from build123d import *

# Parameters (mm, degrees)
BOSS_EXTRUDE1_DEPTH        = 50.8
CUT_EXTRUDE1_REACH         = 65.5
SKETCH2_R                  = 12.7
F_10_32_TAPPED_HOLE1_D     = 4.0386
F_10_32_TAPPED_HOLE1_DEPTH = 6.35
F_10_32_TAPPED_HOLE2_D     = 4.0386
F_10_32_TAPPED_HOLE2_DEPTH = 6.35


with BuildPart() as part:
    # Sketch1 → Boss-Extrude1 (new body)
    with BuildSketch(Plane.XY):
        Polygon((0, 0), (63.5, 0), (63.5, -63.5), (57.15, -63.5), (57.15, -6.35), (0, -6.35), align=None)
    extrude(amount=BOSS_EXTRUDE1_DEPTH)

    # Sketch2 → Cut-Extrude1 (cut, up to next)
    with BuildSketch(Plane(origin=(63.5, 0, 0), x_dir=(0, 0, -1), z_dir=(1, 0, 0)), mode=Mode.PRIVATE) as cut_extrude1_sk1:
        with Locations((-25.4, -31.75)):
            Circle(SKETCH2_R)
    cut_extrude1_tool1 = extrude(cut_extrude1_sk1.sketch, amount=-CUT_EXTRUDE1_REACH, mode=Mode.PRIVATE) & part.part
    add(cut_extrude1_tool1.solids().sort_by_distance((63.5, -31.75, 25.4))[0], mode=Mode.SUBTRACT)

    # #10-32 Tapped Hole1
    with Locations(Plane(origin=(63.5, 0, 0), x_dir=(0, 0, -1), z_dir=(1, 0, 0))):
        with Locations((-34.925, -50.8), (-15.875, -50.8), (-34.925, -12.7), (-15.875, -12.7)):
            Hole(F_10_32_TAPPED_HOLE1_D / 2, depth=F_10_32_TAPPED_HOLE1_DEPTH)

    # #10-32 Tapped Hole2
    with Locations(Plane(origin=(0, 0, 0), x_dir=(1, 0, 0), z_dir=(0, 1, 0))):
        with Locations((47.625, -44.45), (31.75, -38.1), (15.875, -44.45)):
            Hole(F_10_32_TAPPED_HOLE2_D / 2, depth=F_10_32_TAPPED_HOLE2_DEPTH)


solid = part.part
The listing builds one solid part. Answer for the finished solid, in the listing's coordinates (mm). A direction names the side the tool comes from. Round coordinates to 2 decimals unless told otherwise and drop trailing zeros. Order: outer loops, then holes, each group sorted by start corner. A loop starts at its lowest first (then second) coordinate and runs counter-clockwise, first axis right, second up. Notation, with made-up numbers: M 80.25,72 L 118.25,72 A18 ccw 118.25,84 Z; hole C -16.75,9 d3. An arc over 180 degrees is marked long. Answer in a Markdown table with one row per item. Add a question column.
1) The part is cut by section D-D on z = 31. Determine the outline of the cut face in (x, y).
2) Flat-ended cylindrical pins translate along their axes: pin 1 Ø1.5 at (y, z) = (-28, 43.5) entering from -X; pin 2 Ø12 at (x, y) = (20.5, -12) entering from -Z; pin 3 Ø5 at (y, z) = (-38, 30) entering from -X; pin 4 Ø15 at (x, z) = (29, 14.5) entering from -Y. Find the tip coordinate at first contact, or state that the pin passes through.
3) Determine the mould class of faces 3 (the face through (46.539, -3.219, 42.747)), 4 (the face through (58, -17, 50.8)), 5 (the face through (58, -17, 0)), 6 (the face through (60.28, -52.59, 35.86)) for opening direction Z: pulls with the +Z half, pulls with the -Z half, needs draft (parallel to the pull), parting line crosses it, or undercut.
4) Which of the six approach directions +Z, -Z, +X, -X, +Y, -Y give full straight-line access (tool end or side, diameter ignored) to faces 1 (the face through (60.369, -43.017, 19.54)), 2 (the face through (29, -6.35, 25))?
5) The part is cut by section A-A on z = 44.45. Determine the outline of the cut face in (x, y).
6) The part is cut by section C-C on y = -31.75. Determine the outline of the cut face in (x, z).
7) The part is cut by section B-B on x = 59.5. Determine the outline of the cut face in (y, z) (3 decimals).
8) Consider line 1 along Z through (x, y) = (62, -12); line 2 along Y through (x, z) = (50, 43.5); line 3 along X through (y, z) = (-11, 37). Determine where each line is inside the solid, lowest interval first. Write a range as from..to.
Findings below:
| question | item | result |
|---|---|---|
| 1 | outline | M 0,-6.35 L 57.15,-6.35 L 57.15,-20.35 L 63.5,-20.35 L 63.5,0 L 0,0 Z; M 57.15,-63.5 L 63.5,-63.5 L 63.5,-43.15 L 57.15,-43.15 Z |
| 2 | pin 1 | stops at x = 57.15 |
| 2 | pin 2 | stops at z = 0 |
| 2 | pin 3 | passes through |
| 2 | pin 4 | stops at y = -6.35 |
| 3 | face 3 | undercut |
| 3 | face 4 | pulls with the +Z half |
| 3 | face 5 | pulls with the -Z half |
| 3 | face 6 | undercut |
| 4 | face 1 | +X, -X |
| 4 | face 2 | +Z, -Z, -X, -Y |
| 5 | outline | M 0,-6.35 L 13.86,-6.35 L 13.86,0 L 0,0 Z; M 17.89,-6.35 L 45.61,-6.35 L 45.61,0 L 17.89,0 Z; M 49.64,-6.35 L 57.15,-6.35 L 57.15,-63.5 L 63.5,-63.5 L 63.5,0 L 49.64,0 Z |
| 6 | outline | M 57.15,0 L 63.5,0 L 63.5,12.7 L 57.15,12.7 Z; M 57.15,38.1 L 63.5,38.1 L 63.5,50.8 L 57.15,50.8 Z |
| 7 | outline | M -63.5,0 L 0,0 L 0,50.8 L -63.5,50.8 Z; hole C -50.8,15.875 d4.039; hole C -50.8,34.925 d4.039; hole C -31.75,25.4 d25.4; hole C -12.7,15.875 d4.039; hole C -12.7,34.925 d4.039 |
| 8 | line 1 | z = 0..13.98, 17.77..33.03, 36.82..50.8 |
| 8 | line 2 | y = -6.35..0 |
| 8 | line 3 | x = 57.15..63.5 |
